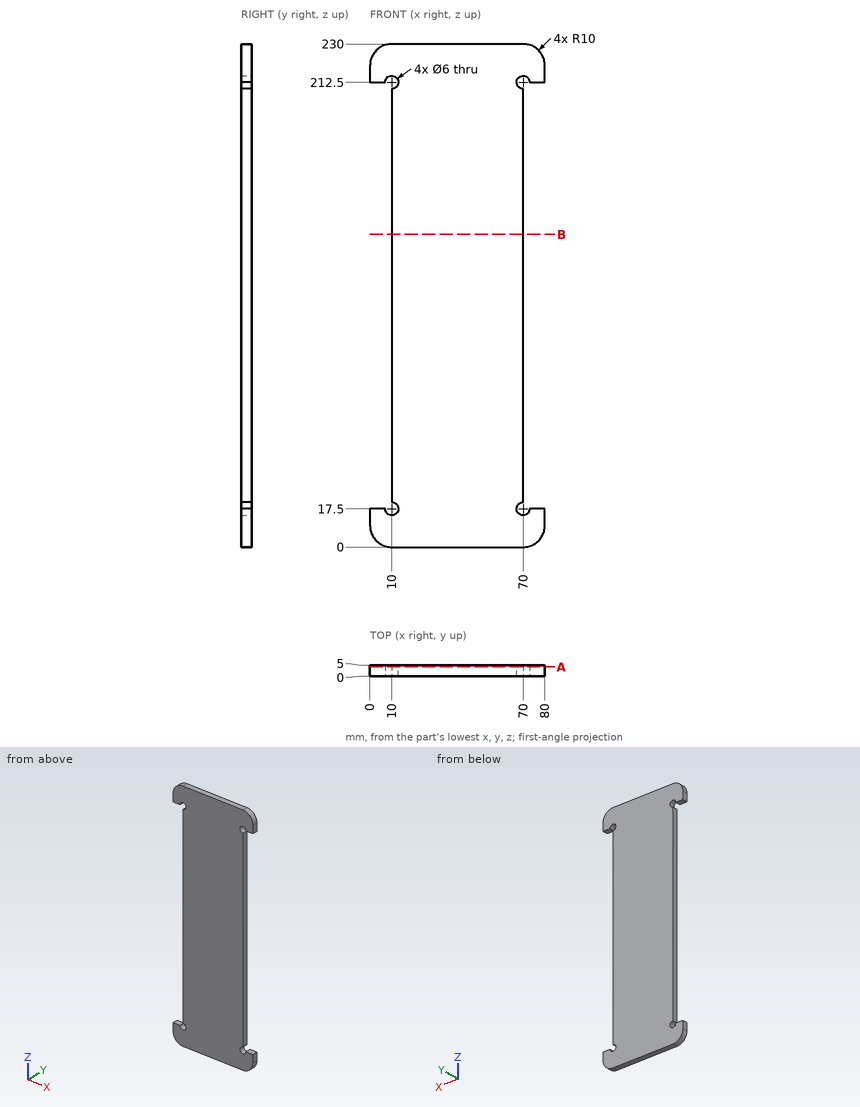
Geometry check sheet. Reference: drawing and pictorial views, mm from the part's lowest x, y, z. Round coordinates to 2 decimals unless told otherwise and drop trailing zeros. Loops run counter-clockwise (first coordinate to the right, second up) from the corner with the lowest first, then second, coordinate; pieces in that order, holes last. Notation, with made-up numbers: (-7, -17) - (49, -17) arc R16 cw to (49, 10) - close; hole circle Ø3 at (78.5, 54.25). An arc over 180 degrees is marked (long way). Write item = value, one per line. Start each with the question number.
Q1. Depth check by flat-ended pin: P1, Ø1, axis at y = 4.5, z = 184.5, coming from the +X side; P2, Ø2.5, axis at x = 3.5, y = 2.5, coming from the +Z side; P3, Ø2.5, axis at y = 3.5, z = 146.5, coming from the -X side. Enter the tip coordinate at first touch or a pass-through.
Q2. Thickness scan on L1, parallel to X at y = 4.5, z = 178.5. Record the ranges inside material, lowest first.
Q3. Section check B-B (z = 143). Record the boundary of the cut face in (x, y).
Q4. Section check A-A (y = 4.2). Record the boundary of the cut face in (x, z), plus the area to 3 significant figures.
Derived:
q1.P1 = 70
q1.P2 = 228.51
q1.P3 = 10
q2.L1 = 10 to 70
q3.outline = (10, 0) - (70, 0) - (70, 5) - (10, 5) - close
q4.outline = (0, 10) arc R10 ccw to (10, 0) - (70, 0) arc R10 ccw to (80, 10) - (80, 17.5) - (73, 17.5) arc R3 cw (long way) to (70, 20.5) - (70, 209.5) arc R3 cw (long way) to (73, 212.5) - (80, 212.5) - (80, 220) arc R10 ccw to (70, 230) - (10, 230) arc R10 ccw to (0, 220) - (0, 212.5) - (7, 212.5) arc R3 cw (long way) to (10, 209.5) - (10, 20.5) arc R3 cw (long way) to (7, 17.5) - (0, 17.5) - close
q4.area = 14,300 mm^2
